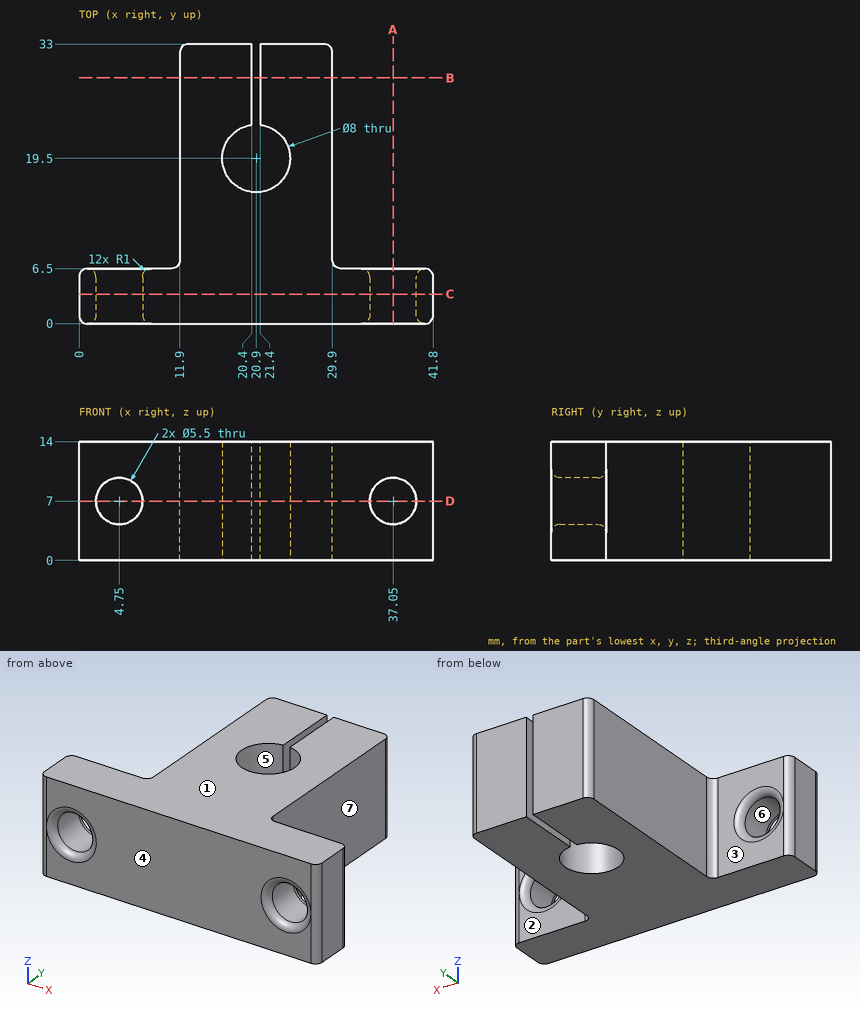
Input: dimensioned drawing with shaded views. Units: mm. Origin: part minimum x, y, z. A direction names the side the tool comes from. Give positions to 0.01 mm unless a question says otherwise; leave off trailing zeros. Write each loop counter-clockwise with the first axis right and the second up, starting at its lowest first coordinate (ties: lowest second). Pieces come first, ordered by that corner, then holes. Notation, with made-up numbers: (1.25, -8.5) - (39.25, -8.5) arc R35 ccw to (39.25, 24.5) - close; hole circle Ø3 at (-33, 78.25). An arc over 180 degrees is marked (long way). Write item = value, one per line. Start each with the question number.
1) Cut plane C-C (y = 3.5). Return loops of the section in (x, z), and give its area (3 significant figures).
2) Draft query along X for the marked faces 4, 5, 6 and 7. Return one class per face: pulls with the +X half, pulls with the -X half, needs draft (parallel to the pull), parting line crosses it, or undercut.
3) Cut plane D-D (z = 7). Give the number of separate pieces and of enclosed holes in the cut face, and give its area (3 significant figures).
4) Pin query (flat end, axial travel): pin 1 (3 mm diameter, centred on y = 26, z = 7, fed in from +X); pin 2 (4 mm diameter, centred on y = 21, z = 10, fed in from -X); pin 3 (5 mm diameter, centred on x = 36.5, z = 4.5, fed in from +Y); pin 4 (5 mm diameter, centred on x = 37.05, z = 7, fed in from +Y). Return the tip coordinate at first contact, or that it passes through.
5) Reachability of the marked faces 1, 2 and 3 from +Z, -Z, +X, -X, +Y, -Y: full face, straight path, thin tool, end or side. Return the list, or none.
6) Cut plane B-B (y = 29). Return loops of the section in (x, z), and give its area (3 significant figures).
7) Cut plane A-A (x = 37.05). Return loops of the section in (y, z).
8) Material intervals for L1, parallel to X at y = 3.9, z = 7; L2, parallel to X at y = 19.5, z = 11.25; L3, parallel to Z at x = 37.05, y = 4.35, sorted ascending. Write a range as [from, to].
Answers follow:
q1.outline = (0, 0) - (41.8, 0) - (41.8, 14) - (0, 14) - close; hole circle Ø5.5 at (4.75, 7); hole circle Ø5.5 at (37.05, 7)
q1.area = 538 mm^2
q2.face_4 = needs draft
q2.face_5 = undercut
q2.face_6 = undercut
q2.face_7 = pulls with the +X half
q3.separate_pieces = 3
q3.enclosed_holes = 0
q3.area = 615 mm^2
q4.pin_1 = 29.9
q4.pin_2 = 11.9
q4.pin_3 = 6.5
q4.pin_4 = through
q5.face_1 = +Z, +X, -X, +Y, -Y
q5.face_2 = +Z, -Z, +X, +Y
q5.face_3 = +Z, -Z, -X, +Y
q6.outline = (11.9, 0) - (20.4, 0) - (20.4, 14) - (11.9, 14) - close; (21.4, 0) - (29.9, 0) - (29.9, 14) - (21.4, 14) - close
q6.area = 238 mm^2
q7.outline = (0, 0) - (6.5, 0) - (6.5, 3.25) arc R1 ccw to (5.5, 4.25) - (1, 4.25) arc R1 ccw to (0, 3.25) - close; (0, 10.75) arc R1 ccw to (1, 9.75) - (5.5, 9.75) arc R1 ccw to (6.5, 10.75) - (6.5, 14) - (0, 14) - close
q8.L1 = [0, 2], [7.5, 34.3], [39.8, 41.8]
q8.L2 = [11.9, 16.9], [24.9, 29.9]
q8.L3 = [0, 4.25], [9.75, 14]
